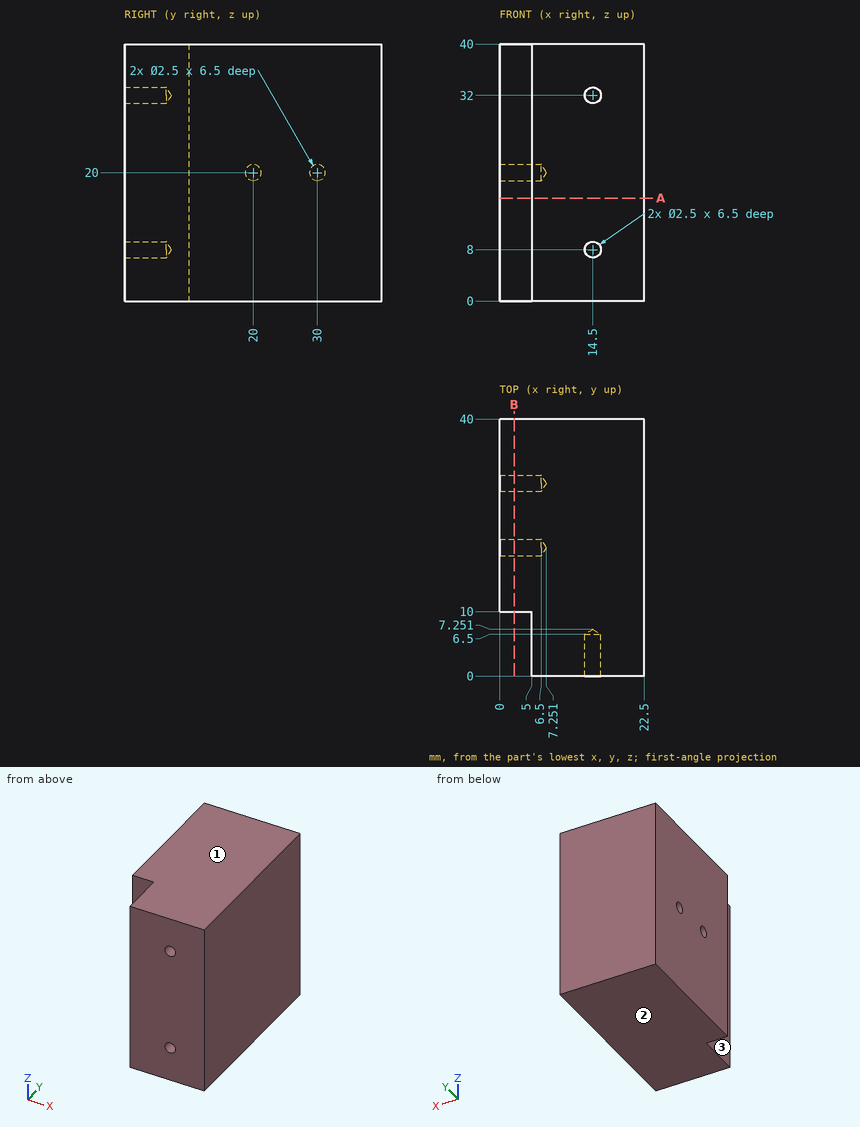
Print and shaded views of the part. All mm, measured from the part's lowest x, y and z. Round coordinates to 2 decimals unless told otherwise and drop trailing zeros. Order: outer loops, then holes, each group sorted by start corner. A loop starts at its lowest first (then second) coordinate and runs counter-clockwise, first axis right, second up.
Q1. Slice it at B-B (x = 2.25). Write the cut outline in (y, z), and give its area (3 significant figures).
Q2. Wall check: L1, parallel to Z at x = 14.5, y = 5.25; L2, parallel to Y at x = 5.25, z = 20; L3, parallel to Y at x = 3, z = 20. Give the ranges that are in metal, low to high.
Q3. Two-plate mould, pull along Z, no slides. Class the marked faces 1, 2 and 3: pulls with the +Z half, pulls with the -Z half, needs draft (parallel to the pull), parting line crosses it, or undercut.
Q4. Drop flat-ended pins along their axis: pin 1 (5 mm diameter, centred on y = 4, z = 23, fed in from -X); pin 2 (1.5 mm diameter, centred on x = 14.5, z = 32, fed in from -Y); pin 3 (1.5 mm diameter, centred on x = 3, z = 19.5, fed in from -Y). Give the stop position or say it passes through.
Q5. Slice it at A-A (z = 16). Write the cut outline in (x, y).
Results below:
1. outline: (10, 0) - (40, 0) - (40, 40) - (10, 40) - close; hole circle Ø2.5 at (20, 20); hole circle Ø2.5 at (30, 20)
1. area: 1,190 mm2
2. L1: z = 0 to 6.75, 9.25 to 30.75, 33.25 to 40
2. L2: y = 0 to 18.75, 21.25 to 28.75, 31.25 to 40
2. L3: y = 10 to 18.75, 21.25 to 28.75, 31.25 to 40
3. face 1: pulls with the +Z half
3. face 2: pulls with the -Z half
3. face 3: needs draft
4. pin 1: stops at x = 5
4. pin 2: stops at y = 6.8
4. pin 3: stops at y = 10
5. outline: (0, 10) - (5, 10) - (5, 0) - (22.5, 0) - (22.5, 40) - (0, 40) - close
